```python
from build123d import *

# Parameters (mm, degrees)
SKETCH_W        = 38
SKETCH_H        = 5
SKETCH_R        = 1.3
PAD_DEPTH       = 12
SKETCH001_R     = 3.33
SKETCH001_R_2   = 1
POCKET_DEPTH    = 5.001
POCKET001_DEPTH = 3


with BuildPart() as part:
    # Sketch → Pad (new body, symmetric)
    with BuildSketch(Plane.XY):
        Rectangle(SKETCH_W, SKETCH_H)
        with Locations((-16.5, 0)):
            Circle(SKETCH_R, mode=Mode.SUBTRACT)
        with Locations((16.5, 0)):
            Circle(SKETCH_R, mode=Mode.SUBTRACT)
    extrude(amount=PAD_DEPTH, both=True)

    # Sketch001 (on Face3 of Pad) → Pocket (cut, through all)
    with BuildSketch(Plane.XZ.offset(2.5)):
        with Locations((0, 3.42)):
            Circle(SKETCH001_R)
        with Locations((7, -6)):
            Circle(SKETCH001_R_2)
        with Locations((13, -6)):
            Circle(SKETCH001_R_2)
        with BuildLine():
            Line((4, -1.7), (-10.4, -1.7))
            ThreePointArc((-10.4, -1.7), (-11.814214, -2.285786), (-12.4, -3.7))
            Line((-12.4, -3.7), (-12.4, -8.9))
            ThreePointArc((-12.4, -8.9), (-11.814214, -10.314214), (-10.4, -10.9))
            Line((-10.4, -10.9), (4, -10.9))
            Line((4, -10.9), (4, -1.7))
        make_face()
        with BuildLine():
            ThreePointArc((-11, 9.6), (-12.6, 8), (-11, 6.4))
            Line((-11, 6.4), (-6, 6.4))
            ThreePointArc((-6, 6.4), (-4.4, 8), (-6, 9.6))
            Line((-11, 9.6), (-6, 9.6))
        make_face()
        with BuildLine():
            ThreePointArc((6, 9.6), (4.4, 8), (6, 6.4))
            Line((6, 6.4), (11, 6.4))
            ThreePointArc((11, 6.4), (12.6, 8), (11, 9.6))
            Line((6, 9.6), (11, 9.6))
        make_face()
    extrude(amount=-POCKET_DEPTH, mode=Mode.SUBTRACT)

    # Sketch002 (on Face23 of Pocket) → Pocket001 (cut)
    with BuildSketch(Plane.XZ.offset(2.5)):
        with BuildLine():
            Line((-12, 11), (12, 11))
            ThreePointArc((15, 8), (14.12132, 10.12132), (12, 11))
            Line((15, 8), (15, -8))
            ThreePointArc((12, -11), (14.12132, -10.12132), (15, -8))
            Line((12, -11), (-12, -11))
            ThreePointArc((-15, -8), (-14.12132, -10.12132), (-12, -11))
            Line((-15, -8), (-15, 8))
            ThreePointArc((-12, 11), (-14.12132, 10.12132), (-15, 8))
        make_face()
    extrude(amount=-POCKET001_DEPTH, mode=Mode.SUBTRACT)


solid = part.part
```
Model file for the job. Use its own axes, mm. A direction names the side the tool comes from. Round coordinates to 2 decimals unless told otherwise and drop trailing zeros. Order: outer loops, then holes, each group sorted by start corner. A loop starts at its lowest first (then second) coordinate and runs counter-clockwise, first axis right, second up. Notation, with made-up numbers: (0.5, 76) -> (24.5, 76) arc R23 cw to (24.5, 93) -> close; hole circle Ø1 at (48.5, -34.75). An arc over 180 degrees is marked (long way). Use one line per item in the form item = value.
Item 1: Cut at B-B, the plane x = -16.5. Write the cut outline in (y, z), and give its area (3 significant figures).
Returned:
outline = (-2.5, -12) -> (-1.3, -12) -> (-1.3, 12) -> (-2.5, 12) -> close; (1.3, -12) -> (2.5, -12) -> (2.5, 12) -> (1.3, 12) -> close
area = 57.6 mm^2
Item 2: Drill centre lines: line 1 (Z direction, x = -10, y = 1.8); line 2 (Z direction, x = 7, y = 2.05); line 3 (Z direction, x = -11.5, y = 0.4). Where is each one in solid material? Low to high.
Returned:
line_1 = -12 to -10.9, -1.7 to 6.4, 9.6 to 12
line_2 = -12 to -7, -5 to 6.4, 9.6 to 12
line_3 = -12 to -11, 11 to 12
Item 3: Pull direction Z, two halves, no side cores. Call faces 1 (the face through (-11.83, 1.49, -10.3)), 2 (the face through (4.4, 1.5, 8)), 3 (the face through (15.2, 0.06, -0.17)): released by +Z, released by -Z, zero draft, split by the parting line, or undercut.
Returned:
face_1 = undercut
face_2 = undercut
face_3 = zero draft
Item 4: Cut at D-D, the plane z = -6. Write the cut outline in (x, y).
Returned:
outline = (-19, -2.5) -> (-15, -2.5) -> (-15, 0.5) -> (-12.4, 0.5) -> (-12.4, 2.5) -> (-19, 2.5) -> close; (4, 0.5) -> (6, 0.5) -> (6, 2.5) -> (4, 2.5) -> close; (8, 0.5) -> (12, 0.5) -> (12, 2.5) -> (8, 2.5) -> close; (14, 0.5) -> (15, 0.5) -> (15, -2.5) -> (19, -2.5) -> (19, 2.5) -> (14, 2.5) -> close; hole circle Ø2.6 at (-16.5, 0); hole circle Ø2.6 at (16.5, 0)
Item 5: Flat gauge pins, fed straight in: pin 1 Ø2 at (x, z) = (11, -4) entering from -Y; pin 2 Ø1.8 at (x, z) = (13, -6) entering from +Y. Where does each tip first touch, or does it go through?
Returned:
pin_1 = 0.5
pin_2 = through
Item 6: Tool access for faces 4 (the face through (15, -1, 0)), 5 (the face through (-3, 1, -1.7)), 6 (the face through (-0.1, -2.5, 11.6)): list every direction of +Z, -Z, +X, -X, +Y, -Y with a clear straight run to the whole face (end or side of a thin tool).
Returned:
face_4 = -Y
face_5 = +Y, -Y
face_6 = +Z, -Z, +X, -X, -Y
Item 7: Cut at A-A, the plane z = 3.42. Write the cut outline in (x, y).
Returned:
outline = (-19, -2.5) -> (-15, -2.5) -> (-15, 0.5) -> (-3.33, 0.5) -> (-3.33, 2.5) -> (-19, 2.5) -> close; (3.33, 0.5) -> (15, 0.5) -> (15, -2.5) -> (19, -2.5) -> (19, 2.5) -> (3.33, 2.5) -> close; hole circle Ø2.6 at (-16.5, 0); hole circle Ø2.6 at (16.5, 0)
Item 8: Cut at C-C, the plane y = -0.5. Write the cut outline in (x, z).
Returned:
outline = (-19, -12) -> (-17.7, -12) -> (-17.7, 12) -> (-19, 12) -> close; (-15.3, -12) -> (15.3, -12) -> (15.3, 12) -> (-15.3, 12) -> close; (17.7, -12) -> (19, -12) -> (19, 12) -> (17.7, 12) -> close; hole (-15, -8) arc R3 ccw to (-12, -11) -> (12, -11) arc R3 ccw to (15, -8) -> (15, 8) arc R3 ccw to (12, 11) -> (-12, 11) arc R3 ccw to (-15, 8) -> close
